from build123d import *

# Parameters (mm, degrees)
F2_DEPTH  = 25.4
F3_DEPTH  = 25.4
F5_DEPTH  = 20.32
F7_DEPTH  = 22.8346
F8_W      = 44.694509
F8_H      = 15.718196
F9_DEPTH  = 17.6276
F11_DEPTH = 11.43


with BuildPart() as f2:
    # F1 (on Top) → F2 (new body)
    with BuildSketch(Plane.XY):
        Polygon((-41.91, 20.32), (-41.91, 0), (-41.91, -20.32), (41.91, -20.32), (41.91, 20.32), align=None)
    extrude(amount=F2_DEPTH)

    # F0 (on Top) → F3 (cut)
    with BuildSketch(Plane.XY):
        Polygon((-35.56, 12.7), (-35.56, 0), (-35.56, -12.7), (35.56, -12.7), (35.56, 12.7), align=None)
    extrude(amount=F3_DEPTH, mode=Mode.SUBTRACT)

    # F4 (on Top) → F5 (cut)
    with BuildSketch(Plane.XY):
        Polygon((-44.768266, 0), (-40.64, 0), (-40.64, -18.796), (40.64, -18.796), (40.64, 18.796), (40.64, 29.692128), (-40.64, 29.692128), (-44.768266, 29.847285), align=None)
    extrude(amount=F5_DEPTH, mode=Mode.SUBTRACT)

    # F6 (on Top) → F7 (cut)
    with BuildSketch(Plane.XY):
        Polygon((39.612409, -11.161779), (39.612409, 0), (39.612409, 11.161779), (39.612409, 23.861779), (35.112143, 23.861779), (35.112143, 11.161779), (35.112143, 0), (35.112143, -11.161779), align=None)
        Polygon((-36.364518, -11.161779), (35.112143, -11.161779), (35.112143, 0), (35.112143, 11.161779), (35.112143, 23.861779), (-37.475668, 23.861779), align=None)
    extrude(amount=F7_DEPTH, mode=Mode.SUBTRACT)

    # F8 (on Top) → F9 (cut)
    with BuildSketch(Plane.XY):
        with Locations((-22.347254, 7.859098)):
            Rectangle(F8_W, F8_H)
    extrude(amount=F9_DEPTH, mode=Mode.SUBTRACT)

    # F10 (on Top) → F11 (cut)
    with BuildSketch(Plane.XY):
        Polygon((-63.650727, 47.761548), (-64.214841, 0), (-64.214841, -44.940986), (66.283256, -44.940986), (66.283256, 49.265854), align=None)
    extrude(amount=F11_DEPTH, mode=Mode.SUBTRACT)


solid = f2.part
Here's how the part is built. I have some questions about the finished solid (model axes, mm). A direction names the side the tool comes from. Round coordinates to 2 decimals unless told otherwise and drop trailing zeros. Order: outer loops, then holes, each group sorted by start corner. A loop starts at its lowest first (then second) coordinate and runs counter-clockwise, first axis right, second up. Notation, with made-up numbers: M -15,-24 L 31,-24 A21 ccw 31,-15 Z; hole C 57,48 d5. An arc over 180 degrees is marked long. Return JSON: item names as keys, results as strings. Group by question number.
1. If we section it at B-B on y = -3: List the corners of the cut face in (x, z) for me.
2. On a 3-axis mill with a long thin cutter (end or side, diameter ignored), from which of +Z, -Z, +X, -X, +Y, -Y can I reach the whole of each face in a straight line? I mean faces 1 (the face through (0, 12.7, 24)), 2 (the face through (0, 20.32, 24)), 3 (the face through (39.612, 4, 22)). Say none if no direction works.
3. If we section it at C-C on z = 16.5: List the corners of the cut face in (x, y) for me, then the cut area to 3 significant figures.
4. If we section it at A-A on x = 24: List the corners of the cut face in (y, z) for me.
5. Please list where these lines run through material, in increasing order: probe 1 along X at (y, z) = (5, 24.5); probe 2 along Y at (x, z) = (6.5, 23); probe 3 along Y at (x, z) = (20.5, 20.5).
6. If we mould it in two halves opening along X, with no side actions, what happens to faces 4 (the face through (-1, 14, 25.4)), 5 (the face through (-40.64, -9, 16)), 6 (the face through (-41.91, -4, 20))? For each: pulls with the +X half, pulls with the -X half, needs draft (parallel to the pull), parting line crosses it, or undercut.
7. I'm going to push flat-ended pins straight in: pin 1 Ø4.5 at (y, z) = (2.5, 14.5) entering from -X; pin 2 Ø1.4 at (x, z) = (-41, 17.5) entering from +Y; pin 3 Ø10 at (x, y) = (-27.5, -5) entering from +Z; pin 4 Ø19.5 at (x, y) = (16.5, -8) entering from -Z. Where does each tip first touch, or does it pass through?
8. If we section it at D-D on y = 3.5: List the corners of the cut face in (x, z) for me, then the cut area to 3 significant figures.
Reply:
{
 "1": {"outline": "M -41.91,11.43 L -40.64,11.43 L -40.64,20.32 L -36.62,20.32 L -36.62,22.83 L -35.56,22.83 L -35.56,25.4 L -41.91,25.4 Z; M 35.56,22.83 L 39.61,22.83 L 39.61,20.32 L 40.64,20.32 L 40.64,11.43 L 41.91,11.43 L 41.91,25.4 L 35.56,25.4 Z"},
 "2": {"face 1": "+Z, -Z", "face 2": "+Z, -Z, +X, -X, +Y", "face 3": "-Z, +Y"},
 "3": {"outline": "M -41.91,-20.32 L 41.91,-20.32 L 41.91,20.32 L 40.64,20.32 L 40.64,-18.8 L -40.64,-18.8 L -40.64,0 L -41.91,0 Z", "area": "201 mm^2"},
 "4": {"outline": "M -20.32,11.43 L -18.8,11.43 L -18.8,20.32 L -12.7,20.32 L -12.7,25.4 L -20.32,25.4 Z; M 12.7,22.83 L 20.32,22.83 L 20.32,25.4 L 12.7,25.4 Z"},
 "5": {"probe 1": "-41.91 to -35.56, 35.56 to 41.91", "probe 2": "-20.32 to -12.7, 12.7 to 20.32", "probe 3": "-20.32 to -12.7"},
 "6": {"face 4": "needs draft", "face 5": "undercut", "face 6": "pulls with the -X half"},
 "7": {"pin 1": "x = 40.64", "pin 2": "y = 0", "pin 3": "through", "pin 4": "z = 20.32"},
 "8": {"outline": "M -41.91,20.32 L -36.83,20.32 L -36.83,22.83 L -35.56,22.83 L -35.56,25.4 L -41.91,25.4 Z; M 35.56,22.83 L 39.61,22.83 L 39.61,20.32 L 40.64,20.32 L 40.64,11.43 L 41.91,11.43 L 41.91,25.4 L 35.56,25.4 Z", "area": "62.4 mm^2"}
}
